```python
from build123d import *

# Parameters (mm, degrees)
ESBO_O1_W              = 230
ESBO_O1_H              = 150
ESBO_O1_R              = 2.5
FLANGE_BASE1_DEPTH     = 2
ARESTA_FLANGE1_DEPTH   = 230
ARESTA_FLANGE1_2_DEPTH = 230
CORTE_EXTRUS_O1_REACH  = 274.044
ESBO_O11_W             = 175.23
ESBO_O11_H             = 135.23


# Read off the part's stored shape, not the designer's step: Aresta-Flange1
# Sheet-metal steps are written as plain solids
with BuildPart() as part:
    # Esboço1 → Flange-base1 (new body)
    with BuildSketch(Plane(origin=(0, 0, 0), x_dir=(1, 0, 0), z_dir=(0, 1, 0))):
        with Locations((115, -75)):
            Rectangle(ESBO_O1_W, ESBO_O1_H)
        with Locations(Location((30, -22.5, 0), (0, 0, 270))):
            Circle(ESBO_O1_R, mode=Mode.SUBTRACT)
        with Locations(Location((30, -127.5, 0), (0, 0, 270))):
            Circle(ESBO_O1_R, mode=Mode.SUBTRACT)
        with Locations(Location((200, -127.5, 0), (0, 0, 270))):
            Circle(ESBO_O1_R, mode=Mode.SUBTRACT)
        with Locations(Location((200, -22.5, 0), (0, 0, 270))):
            Circle(ESBO_O1_R, mode=Mode.SUBTRACT)
    extrude(amount=-FLANGE_BASE1_DEPTH)

    # Aresta-Flange1 outline → Aresta-Flange1 (cut)
    with BuildSketch(Plane.YZ):
        with BuildLine():
            ThreePointArc((-2, 146.414770298), (-1.443395312, 148.069037507), (0, 149.050372696))
            Line((0, 149.050372696), (0, 150))
            Line((0, 150), (-2, 150))
            Line((-2, 150), (-2, 146.414770298))
        make_face()
    extrude(amount=ARESTA_FLANGE1_DEPTH, mode=Mode.SUBTRACT)

    # Aresta-Flange1 2 outline → Aresta-Flange1 2 (add)
    with BuildSketch(Plane.YZ):
        with BuildLine():
            Line((156.884572681, 59.422649731), (2.1049, 148.784735418))
            ThreePointArc((2.1049, 148.784735418), (1.079239772, 149.129835223), (0, 149.050372696))
            Line((0, 149.050372696), (0, 146.414770298))
            ThreePointArc((0, 146.414770298), (0.3683, 147.052684611), (1.1049, 147.052684611))
            Line((1.1049, 147.052684611), (155.884572681, 57.690598923))
            Line((155.884572681, 57.690598923), (156.884572681, 59.422649731))
        make_face()
    extrude(amount=ARESTA_FLANGE1_2_DEPTH)

    # Esboço11 → Corte-extrusão1 (cut, up to next)
    with BuildSketch(Plane(origin=(0, 64.951905284, 112.5), x_dir=(1, 0, 0), z_dir=(0, 0.499999999999998, 0.8660254037844398)), mode=Mode.PRIVATE) as corte_extrus_o1_sk1:
        with Locations((115, 24.177614851)):
            Rectangle(ESBO_O11_W, ESBO_O11_H)
    corte_extrus_o1_tool1 = extrude(corte_extrus_o1_sk1.sketch, amount=-CORTE_EXTRUS_O1_REACH, mode=Mode.PRIVATE) & part.part
    add(corte_extrus_o1_tool1.solids().sort_by_distance((115, 85.890334, 100.411193))[0], mode=Mode.SUBTRACT)


solid = part.part
```
Check sheet for the modelled part. Datum: model origin and axes. Units: mm. A direction names the side the tool comes from. Round coordinates to 2 decimals unless told otherwise and drop trailing zeros. Loops run counter-clockwise (first coordinate to the right, second up) from the corner with the lowest first, then second, coordinate; pieces in that order, holes last. Notation, with made-up numbers: (-30, 70) - (18, 70) arc R32 cw to (18, 97) - close; hole circle Ø8 at (25, -25). An arc over 180 degrees is marked (long way). Answer as a JSON object with one key per item and string values. Group by question number.
Q1. Sectioned sample at C-C, the plane y = 73.5. Enter the section's corners in (x, z) (3 decimals), plus the area to 3 significant figures.
Q2. Scan lines: line 1 along X through (y, z) = (-1.5, 127.5); line 2 along X through (y, z) = (-1, 127); line 3 along Y through (x, z) = (188, 114). Record each from-to range of solid material in increasing order. Write a range as [from, to].
Q3. Sectioned sample at D-D, the plane x = 21. Enter the section's corners in (y, z).
Q4. Mould release check, pull along Z, two halves, no side actions. Record for faces 1 (the face through (202, -1, 129)), 2 (the face through (27.385, 85, 100)), 3 (the face through (113.39, 25.818, 132.785)): released by +Z, released by -Z, zero draft, split by the parting line, or undercut.
Q5. Set-up check for faces 4 (the face through (113.39, 11.787, 143.195)), 5 (the face through (113, 0, 72)): record each of +Z, -Z, +X, -X, +Y, -Y from which the full face is reachable in a straight line by a thin tool's end or side.
Q6. Gauge pin test, flat ends, axial feed: P1, Ø8, axis at x = 200, z = 127.5, coming from the +Y side; P2, Ø12, axis at x = 26.5, y = 128.5, coming from the -Z side; P3, Ø3, axis at x = 132.5, z = 126.5, coming from the +Y side; P4, Ø4, axis at x = 200, z = 22.5, coming from the +Y side. Record the tip position at first contact, or that the pin passes through.
Q7. Sectioned sample at A-A, the plane x = 191. Enter the section's corners in (y, z), plus the area to 3 significant figures.
Q8. Sectioned sample at B-B, the plane z = 99. Enter the section's corners in (x, y) (3 decimals), plus the area to 3 significant figures.
Solution:
{
 "1": {"outline": "(0, 105.255) - (27.385, 105.255) - (27.385, 107.565) - (0, 107.565) - close; (202.615, 105.255) - (230, 105.255) - (230, 107.565) - (202.615, 107.565) - close", "area": "126 mm²"},
 "2": {"line 1": "x = [0, 27.5], [32.5, 197.5], [202.5, 230]", "line 2": "x = [0, 27.55], [32.45, 197.55], [202.45, 230]", "line 3": "y = [-2, 0]"},
 "3": {"outline": "(-2, 0) - (0, 0) - (0, 146.41) arc R0.74 cw to (1.1, 147.05) - (155.88, 57.69) - (156.88, 59.42) - (2.1, 148.78) arc R2.74 ccw to (-2, 146.41) - close"},
 "4": {"face 1": "undercut", "face 2": "zero draft", "face 3": "released by -Z"},
 "5": {"face 4": "+Z, +X, -X, +Y", "face 5": "-Z, +X, -X"},
 "6": {"P1": "stops at y = 44.21", "P2": "stops at z = 70.04", "P3": "stops at y = 0", "P4": "passes through"},
 "7": {"outline": "(-2, 0) - (0, 0) - (0, 146.41) arc R0.74 cw to (1.1, 147.05) - (26.33, 132.49) - (27.33, 134.22) - (2.1, 148.78) arc R2.74 ccw to (-2, 146.41) - close; (143.45, 64.87) - (155.88, 57.69) - (156.88, 59.42) - (144.45, 66.6) - close", "area": "387 mm²"},
 "8": {"outline": "(0, -2) - (230, -2) - (230, 0) - (0, 0) - close; (0, 84.335) - (27.385, 84.335) - (27.385, 88.335) - (0, 88.335) - close; (202.615, 84.335) - (230, 84.335) - (230, 88.335) - (202.615, 88.335) - close", "area": "679 mm²"}
}
